Design review of the part shown in the three views and the two pictorial views. Dimensions are in mm from the part's minimum x, y and z. A direction names the side the tool comes from. Round coordinates to 2 decimals unless told otherwise and drop trailing zeros. Loops run counter-clockwise (first coordinate to the right, second up) from the corner with the lowest first, then second, coordinate; pieces in that order, holes last. Notation, with made-up numbers: (5.5, -35) -> (59.5, -35) arc R25 cw to (59.5, -14) -> close; hole circle Ø11 at (-9, 67.5). An arc over 180 degrees is marked (long way). Use a Markdown table: item, result. Add a question column.
1) Consider section D-D on x = 14.5. Give the boundary of the cut face in (y, z), plus the area to 3 significant figures.
2) Mouldability with a two-part tool opening along Y and no side actions: class the marked faces 1, 2 and 3 as released by +Y, released by -Y, zero draft, split by the parting line, or undercut.
3) Insertion check: pin 1 (0.8 mm diameter, centred on x = 33.5, z = 1.5, fed in from -Y); pin 2 (1.6 mm diameter, centred on y = 2.5, z = 9, fed in from -X); pin 3 (3 mm diameter, centred on x = 17.5, z = 6, fed in from -Y); pin 4 (5 mm diameter, centred on x = 24, z = 7, fed in from +Y). Each pin has a flat end and moves straight along its axis. Give the tip position at first contact, or say it passes through.
4) For the marked faces 4, 5 and 6, list the 3-axis set-ups (+Z, -Z, +X, -X, +Y, -Y) from which the entire face can be reached by the end or side of a thin tool; tool diameter is ignored.
5) Consider section B-B on z = 13.75. State how many separate pieces and enclosed holes the cut face has, plus the area to 3 significant figures.
6) Wall thickness on probe 1 along Z at (x, y) = (4.5, 6.5); probe 2 along X at (y, z) = (4, 13.5); probe 3 along X at (y, z) = (5.5, 7.75): over which ranges is each line inside the solid? List them lowest first.
7) Consider section A-A on x = 10. Give the boundary of the cut face in (y, z), plus the area to 3 significant figures.
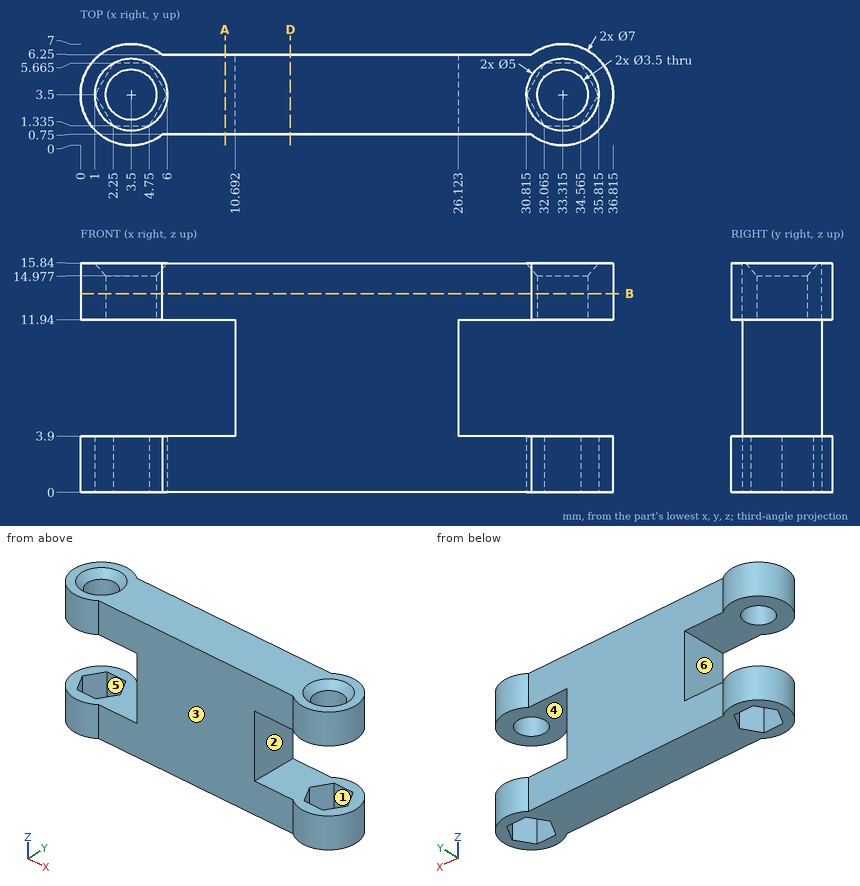
Result set:
| question | item | result |
|---|---|---|
| 1 | outline | (0.75, 0) -> (6.25, 0) -> (6.25, 15.84) -> (0.75, 15.84) -> close |
| 1 | area | 87.1 mm2 |
| 2 | face 1 | undercut |
| 2 | face 2 | zero draft |
| 2 | face 3 | released by -Y |
| 3 | pin 1 | y = 0 |
| 3 | pin 2 | x = 10.69 |
| 3 | pin 3 | y = 0.75 |
| 3 | pin 4 | y = 6.25 |
| 4 | face 4 | +X, +Y, -Y |
| 4 | face 5 | -Z |
| 4 | face 6 | -X, +Y, -Y |
| 5 | separate pieces | 1 |
| 5 | enclosed holes | 2 |
| 5 | area | 188 mm2 |
| 6 | probe 1 | 0 to 3.9, 11.94 to 15.84 |
| 6 | probe 2 | 0.04 to 1.82, 5.18 to 31.64, 34.99 to 36.78 |
| 6 | probe 3 | 10.69 to 26.12 |
| 7 | outline | (0.75, 0) -> (6.25, 0) -> (6.25, 3.9) -> (0.75, 3.9) -> close; (0.75, 11.94) -> (6.25, 11.94) -> (6.25, 15.84) -> (0.75, 15.84) -> close |
| 7 | area | 42.9 mm2 |
